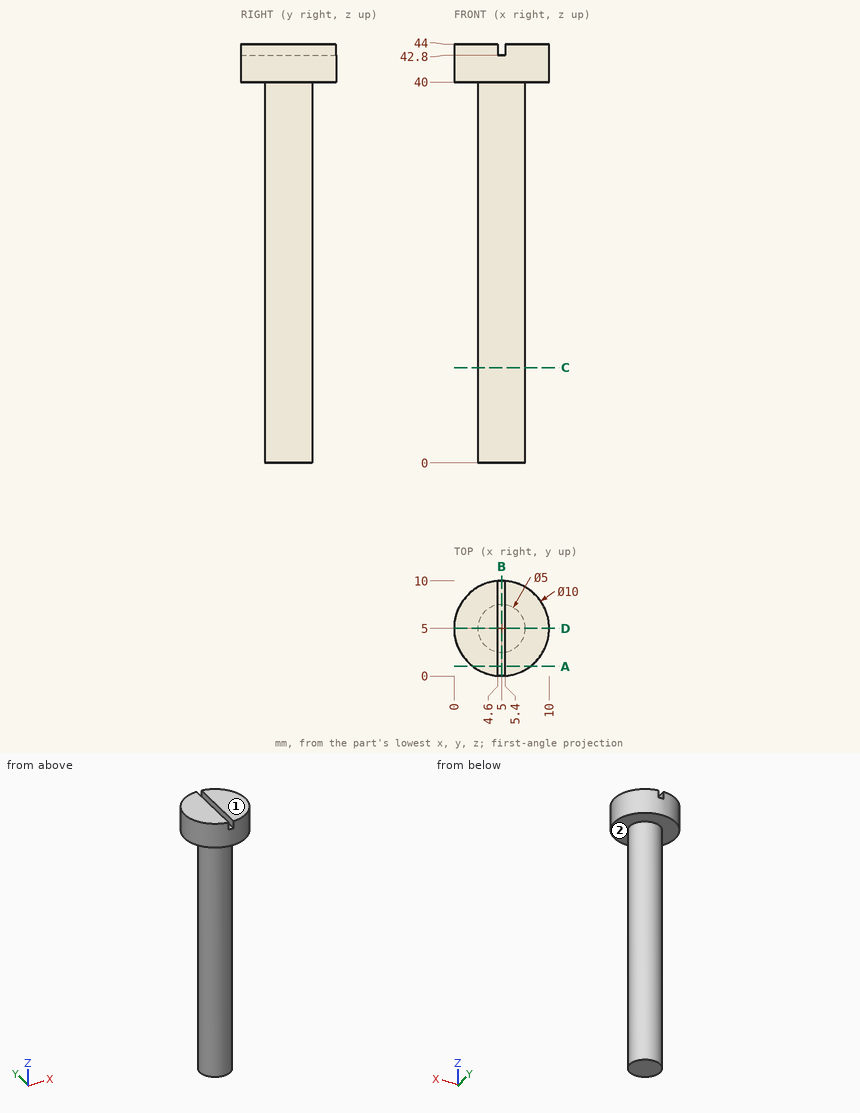
Input: dimensioned drawing with shaded views. Units: mm. Origin: part minimum x, y, z. A direction names the side the tool comes from. Coordinates: 2 decimals unless noted, no trailing zeros. Order: outer loops, then holes, each group sorted by start corner. A loop starts at its lowest first (then second) coordinate and runs counter-clockwise, first axis right, second up. Notation, with made-up numbers: M 67,-32.75 L 81,-32.75 A8 ccw 81,-23.75 Z; hole C 85,80.25 d6. An arc over 180 degrees is marked long. Write each question's results on one line, items separated by ' | '. Start each with the question number.
Item 1: First-contact query: pin 1 Ø3 at (x, z) = (1.5, 30.5) entering from +Y; pin 2 Ø0.6 at (y, z) = (5.5, 43.5) entering from -X; pin 3 Ø1 at (x, z) = (5.5, 13) entering from +Y. Flat tips, straight axial feed; report the tip coordinate or a pass-through.
Item 2: Cut plane C-C (z = 10). Return loops of the section in (x, y).
Item 3: Line query: probe 1 along Z at (x, y) = (3.25, 7.75); probe 2 along Y at (x, z) = (5, 24.5); probe 3 along X at (y, z) = (5.5, 27). Output: solid intervals per line, ascending.
Item 4: Set-up query: the marked faces 1 and 2. Return all of +Z, -Z, +X, -X, +Y, -Y with unobstructed straight access to the full face (end or side cutting, diameter ignored); none if empty.
Item 5: Cut plane D-D (y = 5). Return loops of the section in (x, z).
Item 6: Cut plane A-A (y = 1). Return loops of the section in (x, z).
Item 7: Cut plane B-B (x = 5). Return loops of the section in (y, z), and give its area (3 significant figures).
Checked values:
1) pin 1: stops at y = 6.5 | pin 2: stops at x = 0 | pin 3: stops at y = 7.5
2) outline: C 5,5 d5
3) probe 1: z = 40 to 44 | probe 2: y = 2.5 to 7.5 | probe 3: x = 2.55 to 7.45
4) face 1: +Z, +X, -X, +Y, -Y | face 2: -Z
5) outline: M 0,40 L 2.5,40 L 2.5,0 L 7.5,0 L 7.5,40 L 10,40 L 10,44 L 5.4,44 L 5.4,42.8 L 4.6,42.8 L 4.6,44 L 0,44 Z
6) outline: M 2,40 L 8,40 L 8,44 L 5.4,44 L 5.4,42.8 L 4.6,42.8 L 4.6,44 L 2,44 Z
7) outline: M 0,40 L 2.5,40 L 2.5,0 L 7.5,0 L 7.5,40 L 10,40 L 10,42.8 L 0,42.8 Z | area: 228 mm2
